```python
from build123d import *

# Parameters (mm, degrees)
SKETCH1_R            = 39
SKETCH1_R_2          = 26.5
BOSS_EXTRUDE1_DEPTH  = 2.25
SKETCH3_W            = 50
SKETCH3_H            = 51.5
BOSS_EXTRUDE2_DEPTH  = 2.25
BOSS_EXTRUDE4_DEPTH  = 2.25
SKETCH2_R            = 2.75
CUT_EXTRUDE1_DEPTH   = 3.25
CIRPATTERN1_COUNT    = 6
CUT_EXTRUDE2_START   = -5.5
SKETCH5_R            = 2.25
CUT_EXTRUDE2_DEPTH   = 6.5
LPATTERN1_COUNT      = 2
LPATTERN1_PITCH      = 15
LPATTERN1_COUNT_DIR2 = 2
LPATTERN1_PITCH_DIR2 = 10
LPATTERN2_COUNT      = 2
LPATTERN2_PITCH      = 15
LPATTERN2_COUNT_DIR2 = 2
LPATTERN2_PITCH_DIR2 = 10
CUT_EXTRUDE3_START   = -5.5
SKETCH7_R            = 3.25
CUT_EXTRUDE3_DEPTH   = 6.5
LPATTERN3_COUNT      = 3
LPATTERN3_PITCH      = 20
SKETCH8_R            = 3.25
CUT_EXTRUDE4_DEPTH   = 10
LPATTERN4_COUNT      = 4
LPATTERN4_PITCH      = 20


with BuildPart() as part:
    # Sketch1 → Boss-Extrude1 (new body, symmetric)
    with BuildSketch(Plane(origin=(0, 0, 0), x_dir=(1, 0, 0), z_dir=(0, 1, 0))):
        Circle(SKETCH1_R)
        Circle(SKETCH1_R_2, mode=Mode.SUBTRACT)
    extrude(amount=BOSS_EXTRUDE1_DEPTH, both=True)

    # Sketch3 → Boss-Extrude2 (add, symmetric)
    with BuildSketch(Plane(origin=(0, 0, 0), x_dir=(1, 0, 0), z_dir=(0, 1, 0))):
        with Locations((0, 52.25)):
            Rectangle(SKETCH3_W, SKETCH3_H)
    extrude(amount=BOSS_EXTRUDE2_DEPTH, both=True)

    # Sketch6 → Boss-Extrude4 (add, symmetric)
    with BuildSketch(Plane(origin=(0, 0, 0), x_dir=(1, 0, 0), z_dir=(0, 1, 0))):
        Polygon((-35, 166.5), (-35, 26.5), (-39, 0), (-14.981514186, 26.5), (16.520833333, 26.5), (39, 0), (35, 26.5), (35, 166.5), align=None)
    extrude(amount=BOSS_EXTRUDE4_DEPTH, both=True)

    # Sketch2 → Cut-Extrude1 (cut, symmetric)
    with BuildSketch(Plane(origin=(0, 0, 0), x_dir=(1, 0, 0), z_dir=(0, 1, 0))):
        with Locations((0, 32.5)):
            Circle(SKETCH2_R)
    cut_extrude1 = extrude(amount=CUT_EXTRUDE1_DEPTH, both=True, mode=Mode.SUBTRACT)

    # CirPattern1: Cut-Extrude1 ×6 about axis
    cirpattern1_axis = Axis((0, 0, 0), (0, 1, 0))
    for i in range(1, CIRPATTERN1_COUNT):
        add(cut_extrude1.rotate(cirpattern1_axis, i * 360 / CIRPATTERN1_COUNT), mode=Mode.SUBTRACT)

    # Sketch5 → Cut-Extrude2 (cut)
    with BuildSketch(Plane(origin=(0, 2.25, 0), x_dir=(1, 0, 0), z_dir=(0, 1, 0)).offset(CUT_EXTRUDE2_START)):
        with Locations((0, 73)):
            Circle(SKETCH5_R)
    cut_extrude2 = extrude(amount=CUT_EXTRUDE2_DEPTH, mode=Mode.SUBTRACT)

    # LPattern1: Cut-Extrude2 2 × 2
    with Locations(*[(i * LPATTERN1_PITCH, 0, j * LPATTERN1_PITCH_DIR2) for i in range(LPATTERN1_COUNT) for j in range(LPATTERN1_COUNT_DIR2) if (i, j) != (0, 0)]):
        add(cut_extrude2, mode=Mode.SUBTRACT)

    # LPattern2: Cut-Extrude2 2 × 2
    with Locations(*[(-i * LPATTERN2_PITCH, 0, j * LPATTERN2_PITCH_DIR2) for i in range(LPATTERN2_COUNT) for j in range(LPATTERN2_COUNT_DIR2) if (i, j) != (0, 0)]):
        add(cut_extrude2, mode=Mode.SUBTRACT)

    # Sketch7 → Cut-Extrude3 (cut)
    with BuildSketch(Plane(origin=(0, 2.25, 0), x_dir=(1, 0, 0), z_dir=(0, 1, 0)).offset(CUT_EXTRUDE3_START)):
        with Locations((-15, 146.5)):
            Circle(SKETCH7_R)
        with Locations((15, 146.5)):
            Circle(SKETCH7_R)
    cut_extrude3 = extrude(amount=CUT_EXTRUDE3_DEPTH, mode=Mode.SUBTRACT)

    # LPattern3: Cut-Extrude3 ×3
    with Locations(*[(0, 0, i * LPATTERN3_PITCH) for i in range(1, LPATTERN3_COUNT)]):
        add(cut_extrude3, mode=Mode.SUBTRACT)

    # Sketch8 → Cut-Extrude4 (cut)
    with BuildSketch(Plane(origin=(0, 2.25, 0), x_dir=(1, 0, 0), z_dir=(0, 1, 0))):
        with Locations((0, 146.5)):
            Circle(SKETCH8_R)
    cut_extrude4 = extrude(amount=-CUT_EXTRUDE4_DEPTH, mode=Mode.SUBTRACT)

    # LPattern4: Cut-Extrude4 ×4
    with Locations(*[(0, 0, i * LPATTERN4_PITCH) for i in range(1, LPATTERN4_COUNT)]):
        add(cut_extrude4, mode=Mode.SUBTRACT)


solid = part.part
```
Work out the finished part from the listing and answer in its coordinate system (mm). A direction names the side the tool comes from. Round coordinates to 2 decimals unless told otherwise and drop trailing zeros. Order: outer loops, then holes, each group sorted by start corner. A loop starts at its lowest first (then second) coordinate and runs counter-clockwise, first axis right, second up.
Q1. Given pin 1 Ø2 at (y, z) = (0, -91) entering from -X, flat-ended and moving along its own axis, determine where the tip first touches the part or whether it passes through.
Solution:
pin 1: stops at x = -35
Q2. A cutting plane is placed at A-A, the plane z = 0. Determine the outline of the cut face in (x, y), then the cut area to 4 significant figures.
Solution:
outline: (-39, -2.25) - (-26.5, -2.25) - (-26.5, 2.25) - (-39, 2.25) - close; (26.5, -2.25) - (39, -2.25) - (39, 2.25) - (26.5, 2.25) - close
area: 112.5 mm2
Q3. A cutting plane is placed at B-B, the plane z = -126.5. Determine the outline of the cut face in (x, y).
Solution:
outline: (-35, -2.25) - (-18.25, -2.25) - (-18.25, 2.25) - (-35, 2.25) - close; (-11.75, -2.25) - (-3.25, -2.25) - (-3.25, 2.25) - (-11.75, 2.25) - close; (3.25, -2.25) - (11.75, -2.25) - (11.75, 2.25) - (3.25, 2.25) - close; (18.25, -2.25) - (35, -2.25) - (35, 2.25) - (18.25, 2.25) - close
Q4. A tool of negligible diameter and unlimited length cuts with its end or side. For faces 5 (the flat face through (35, 0, -96)), 6 (the cylindrical face through (-0.358, 0.031, -35.227)), from which of +Z, -Z, +X, -X, +Y, -Y can it reach the whole face along a straight path? Write none if from no direction.
Solution:
face 5: -Z, +X, +Y, -Y
face 6: +Y, -Y
Q5. The mould has two halves that part along X. Classify faces 1 (the flat face through (8, -2.25, -65)), 2 (the flat face through (36.147, 0.031, -18.901)), 3 (the cylindrical face through (25.523, 0.031, -15.424)), 4 (the cylindrical face through (16.5, -0.031, -143.617)): pulls with the +X half, pulls with the -X half, needs draft (parallel to the pull), parting line crosses it, or undercut.
Solution:
face 1: needs draft
face 2: pulls with the +X half
face 3: undercut
face 4: undercut
Q6. A cutting plane is placed at C-C, the plane x = -15. Determine the outline of the cut face in (y, z), then the cut area to 3 significant figures.
Solution:
outline: (-2.25, -166.5) - (2.25, -166.5) - (2.25, -149.75) - (-2.25, -149.75) - close; (-2.25, -143.25) - (2.25, -143.25) - (2.25, -129.75) - (-2.25, -129.75) - close; (-2.25, -123.25) - (2.25, -123.25) - (2.25, -109.75) - (-2.25, -109.75) - close; (-2.25, -103.25) - (2.25, -103.25) - (2.25, -75.25) - (-2.25, -75.25) - close; (-2.25, -70.75) - (2.25, -70.75) - (2.25, -65.25) - (-2.25, -65.25) - close; (-2.25, -60.75) - (2.25, -60.75) - (2.25, -21.85) - (-2.25, -21.85) - close; (-2.25, 21.85) - (2.25, 21.85) - (2.25, 36) - (-2.25, 36) - close
area: 586 mm2
Q7. Find the intervals of material crossed by line 1 along X through (y, z) = (-0.15, -107); line 2 along Z through (x, y) = (28.5, 1); line 3 along Z through (x, y) = (29, 1.45), in increasing order.
Solution:
line 1: x = -35 to -18.21, -11.79 to -3.21, 3.21 to 11.79, 18.21 to 35
line 2: z = -166.5 to -18.98, -13.52 to 13.52, 18.98 to 26.62
line 3: z = -166.5 to -18.86, -13.64 to 13.64, 18.86 to 26.08
Q8. A cutting plane is placed at D-D, the plane y = -0.3. Count the separate pieces of the cut face and the enclosed holes in it, then the cut area to 3 significant figures.
Solution:
separate pieces: 1
enclosed holes: 23
area: 11,400 mm2
